```python
from build123d import *

# Parameters (mm, degrees)
PAD_DEPTH       = 1.27
POCKET_DEPTH    = 0.635
SKETCH002_R     = 1.905
POCKET001_DEPTH = 5.08
PAD001_DEPTH    = 5.08
SKETCH005_W     = 33.528
SKETCH005_H     = 0.6604
POCKET002_DEPTH = 33.02
SKETCH006_W     = 33.528
SKETCH006_H     = 27.94
POCKET003_DEPTH = 2.54
POCKET004_DEPTH = 0.254


with BuildPart() as part:
    # Sketch → Pad (new body)
    with BuildSketch(Plane.XY):
        with BuildLine():
            Line((-15.24, 0), (15.24, 0))
            ThreePointArc((15.24, 0), (17.036051, 0.743949), (17.78, 2.54))
            Line((17.78, 2.54), (17.78, 50.8))
            ThreePointArc((17.78, 50.8), (17.036051, 52.596051), (15.24, 53.34))
            Line((15.24, 53.34), (-15.24, 53.34))
            ThreePointArc((-15.24, 53.34), (-17.036051, 52.596051), (-17.78, 50.8))
            Line((-17.78, 2.54), (-17.78, 50.8))
            ThreePointArc((-17.78, 2.54), (-17.036051, 0.743949), (-15.24, 0))
        make_face()
    extrude(amount=PAD_DEPTH)

    # Sketch001 (on Face9 of Pad) → Pocket (cut)
    with BuildSketch(Plane(origin=(0, 0, 0), x_dir=(1, 0, 0), z_dir=(0, 0, -1))):
        with BuildLine():
            Line((-12.7, -2.54), (12.7, -2.54))
            ThreePointArc((13.97, -3.81), (13.598026, -2.911974), (12.7, -2.54))
            Line((13.97, -3.81), (13.97, -31.75))
            ThreePointArc((12.7, -33.02), (13.598026, -32.648026), (13.97, -31.75))
            Line((12.7, -33.02), (-12.7, -33.02))
            ThreePointArc((-13.97, -31.75), (-13.598026, -32.648026), (-12.7, -33.02))
            Line((-13.97, -3.81), (-13.97, -31.75))
            ThreePointArc((-12.7, -2.54), (-13.598026, -2.911974), (-13.97, -3.81))
        make_face()
    extrude(amount=-POCKET_DEPTH, mode=Mode.SUBTRACT)

    # Sketch002 (on Face4 of Pocket) → Pocket001 (cut)
    with BuildSketch(Plane(origin=(0, 0, 0), x_dir=(1, 0, 0), z_dir=(0, 0, -1))):
        with Locations((0, -36.068)):
            Circle(SKETCH002_R)
        with Locations((8.382, -36.068)):
            Circle(SKETCH002_R)
        with Locations((-8.382, -36.068)):
            Circle(SKETCH002_R)
    extrude(amount=-POCKET001_DEPTH, mode=Mode.SUBTRACT)

    # Sketch004 (on Face5 of Pocket001) → Pad001 (join)
    with BuildSketch(Plane.XY.offset(1.27)):
        with BuildLine():
            Line((-15.24, 0), (15.24, 0))
            ThreePointArc((15.24, 0), (17.036051, 0.743949), (17.78, 2.54))
            Line((17.78, 34.29), (17.78, 2.54))
            Line((17.78, 34.29), (14.859, 34.29))
            ThreePointArc((14.859, 34.29), (14.409987, 34.104013), (14.224, 33.655))
            Line((14.224, 33.655), (14.224, 3.81))
            ThreePointArc((11.684, 1.27), (13.480051, 2.013949), (14.224, 3.81))
            Line((11.684, 1.27), (-11.684, 1.27))
            ThreePointArc((-14.224, 3.81), (-13.480051, 2.013949), (-11.684, 1.27))
            Line((-14.224, 3.81), (-14.224, 33.655))
            ThreePointArc((-14.224, 33.655), (-14.409987, 34.104013), (-14.859, 34.29))
            Line((-17.78, 34.29), (-14.859, 34.29))
            Line((-17.78, 2.54), (-17.78, 34.29))
            ThreePointArc((-17.78, 2.54), (-17.036051, 0.743949), (-15.24, 0))
        make_face()
    extrude(amount=PAD001_DEPTH)

    # Sketch005 (on Face27 of Pad001) → Pocket002 (cut)
    with BuildSketch(Plane(origin=(0, 34.29, 0), x_dir=(-1, 0, 0), z_dir=(0, 1, 0))):
        with Locations((0, 4.1402)):
            Rectangle(SKETCH005_W, SKETCH005_H)
    extrude(amount=-POCKET002_DEPTH, mode=Mode.SUBTRACT)

    # Sketch006 (on Face25 of Pocket002) → Pocket003 (cut)
    with BuildSketch(Plane.XY.offset(6.35)):
        with Locations((0, 20.32)):
            Rectangle(SKETCH006_W, SKETCH006_H)
    extrude(amount=-POCKET003_DEPTH, mode=Mode.SUBTRACT)

    # Sketch007 (on Face8 of Pocket003) → Pocket004 (cut)
    with BuildSketch(Plane.XY.offset(1.27)):
        with BuildLine():
            ThreePointArc((-8.382, 39.878), (-12.192, 36.068), (-8.382, 32.258))
            Line((-8.382, 32.258), (8.382, 32.258))
            ThreePointArc((8.382, 32.258), (12.192, 36.068), (8.382, 39.878))
            Line((8.382, 39.878), (-8.382, 39.878))
        make_face()
    extrude(amount=-POCKET004_DEPTH, mode=Mode.SUBTRACT)


solid = part.part
```
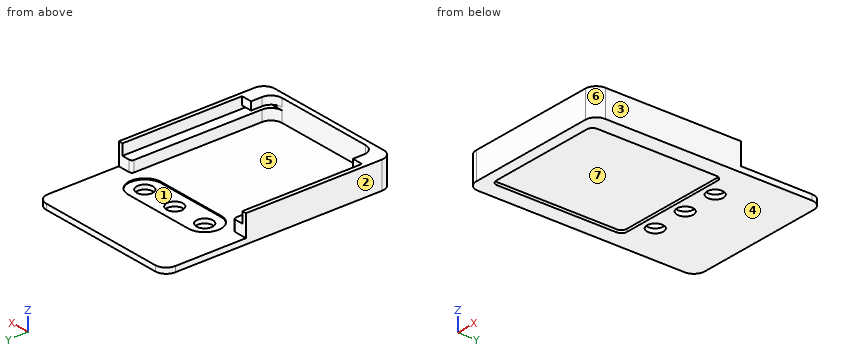
Geometry: final body of the model. Coordinates: model frame, mm. Face numbers are marked on the shaded views. A direction names the side the tool comes from. Give positions to 0.01 mm unless a question says otherwise; leave off trailing zeros. Loops run counter-clockwise (first coordinate to the right, second up) from the corner with the lowest first, then second, coordinate; pieces in that order, holes last. Notation, with made-up numbers: (49.5, 51.25) - (108.5, 51.25) arc R14 ccw to (108.5, 57.25) - close; hole circle Ø11 at (-22, 63). An arc over 180 degrees is marked (long way). Answer as CSV lines item,"result". Start each with the question number.
(1) Section query D-D (y = 43). Output: boundary loops of the cut face in (x, z), and give its area (3 significant figures).
(2) Section query C-C (x = -4). Output: boundary loops of the cut face in (y, z) (3 decimals).
(3) Pin query (flat end, axial travel): P1, Ø3, axis at x = 0, y = 36.068, coming from the -Z side; P2, Ø1.5, axis at x = -16, z = 4, coming from the +Y side; P3, Ø1, axis at x = -1.5, z = 2.5, coming from the +Y side; P4, Ø8, axis at x = 1.5, y = 37.5, coming from the +Z side. Return the tip coordinate at first contact, or that it passes through.
(4) Mould query, pull axis X, two halves, no side actions, for the marked faces 1, 2, 3 and 4. Classes: +X half, -X half, draft (parallel to the pull), parting line (faces both ways), or undercut.
(5) Section query B-B (z = 2.25). Output: boundary loops of the cut face in (x, y) (3 decimals), and give its area (3 significant figures).
(6) Reachability of the marked faces 5, 6 and 7 from +Z, -Z, +X, -X, +Y, -Y: full face, straight path, thin tool, end or side. Return the list, or none.
(7) Section query A-A (x = 0). Output: boundary loops of the cut face in (y, z) (3 decimals).
(8) Ray query, line 1 along X through (y, z) = (29, 3.75); line 2 along X through (y, z) = (14, 0.5); line 3 along Z through (x, y) = (-1, 17.5) (3 decimals). Return the intervals inside material, ascending. Write a range as [from, to].
Worked answers:
1,outline,"(-17.78, 0) - (17.78, 0) - (17.78, 1.27) - (-17.78, 1.27) - close"
1,area,"45.2 mm^2"
2,outline,"(0, 0) - (2.54, 0) - (2.54, 0.635) - (33.02, 0.635) - (33.02, 0) - (53.34, 0) - (53.34, 1.27) - (39.878, 1.27) - (39.878, 1.016) - (32.258, 1.016) - (32.258, 1.27) - (1.27, 1.27) - (1.27, 6.35) - (0, 6.35) - close"
3,P1,"passes through"
3,P2,"stops at y = 34.29"
3,P3,"stops at y = 1.27"
3,P4,"stops at z = 1.27"
4,face 1,"undercut"
4,face 2,"-X half"
4,face 3,"+X half"
4,face 4,"draft"
5,outline,"(-17.78, 2.54) arc R2.54 ccw to (-15.24, 0) - (15.24, 0) arc R2.54 ccw to (17.78, 2.54) - (17.78, 34.29) - (14.859, 34.29) arc R0.635 ccw to (14.224, 33.655) - (14.224, 3.81) arc R2.54 cw to (11.684, 1.27) - (-11.684, 1.27) arc R2.54 cw to (-14.224, 3.81) - (-14.224, 33.655) arc R0.635 ccw to (-14.859, 34.29) - (-17.78, 34.29) - close"
5,area,"280 mm^2"
6,face 5,"+Z, +Y"
6,face 6,"+Z, -Z, +X, -Y"
6,face 7,"-Z"
7,outline,"(0, 0) - (2.54, 0) - (2.54, 0.635) - (33.02, 0.635) - (33.02, 0) - (34.163, 0) - (34.163, 1.016) - (32.258, 1.016) - (32.258, 1.27) - (1.27, 1.27) - (1.27, 6.35) - (0, 6.35) - close; (37.973, 0) - (53.34, 0) - (53.34, 1.27) - (39.878, 1.27) - (39.878, 1.016) - (37.973, 1.016) - close"
8,line 1,"x = [-17.78, -14.22], [14.22, 17.78]"
8,line 2,"x = [-17.78, -13.97], [13.97, 17.78]"
8,line 3,"z = [0.635, 1.27]"
